from build123d import *

# Parameters (mm, degrees)
F1_DEPTH = 2.54
F2_COUNT = 6
F4_R     = 6.35
F5_DEPTH = 0.508


# Not quite as in the source:
# - a feature names something its author has since deleted; it is built from what else it names


with BuildPart() as f1:
    # F0 (on Top) → F1 (new body)
    with BuildSketch(Plane.XY):
        with BuildLine():
            Line((11.3864204897, -39.6875), (22.9135888085, -39.6875))
            Line((22.9135888085, -39.6875), (0, 0))
            Line((0, 0), (-22.9135888085, -39.6875))
            Line((-22.9135888085, -39.6875), (-11.3864204897, -39.6875))
            ThreePointArc((-11.3864204897, -39.6875), (-10.9170896872, -39.3739031836), (-11.0272102448, -38.8202897552))
            Line((-11.0272102448, -38.8202897552), (-11.8327897552, -38.0147102448))
            ThreePointArc((-11.8327897552, -38.0147102448), (-11.9429103128, -37.4610968164), (-11.4735795103, -37.1475))
            Line((-11.4735795103, -37.1475), (-1.905, -37.1475))
            ThreePointArc((-1.905, -37.1475), (-0.5579615818, -37.7054615818), (0, -39.0525))
            Line((0, -39.0525), (0, -39.6875))
            Line((0, -39.6875), (11.3864204897, -39.6875))
        make_face()
        with BuildLine():
            ThreePointArc((11.0272102448, -40.5547102448), (10.9170896872, -40.0010968164), (11.3864204897, -39.6875))
            Line((11.3864204897, -39.6875), (0, -39.6875))
            Line((0, -39.6875), (0, -40.3225))
            ThreePointArc((0, -40.3225), (0.5579615818, -41.6695384182), (1.905, -42.2275))
            Line((1.905, -42.2275), (11.4735795103, -42.2275))
            ThreePointArc((11.4735795103, -42.2275), (11.9429103128, -41.9139031836), (11.8327897552, -41.3602897552))
            Line((11.8327897552, -41.3602897552), (11.0272102448, -40.5547102448))
        make_face()
    extrude(amount=F1_DEPTH)


with BuildPart() as f2_1:
    # F2: instance of F1
    add(f1.part.rotate(Axis((0, 0, 1.27), (0, 0, -1)), 1 * 360 / F2_COUNT))


with BuildPart() as f2_2:
    # F2: instance of F1
    add(f1.part.rotate(Axis((0, 0, 1.27), (0, 0, -1)), 2 * 360 / F2_COUNT))


with BuildPart() as f2_3:
    # F2: instance of F1
    add(f1.part.rotate(Axis((0, 0, 1.27), (0, 0, -1)), 3 * 360 / F2_COUNT))


with BuildPart() as f2_4:
    # F2: instance of F1
    add(f1.part.rotate(Axis((0, 0, 1.27), (0, 0, -1)), 4 * 360 / F2_COUNT))


with BuildPart() as f2_5:
    # F2: instance of F1
    add(f1.part.rotate(Axis((0, 0, 1.27), (0, 0, -1)), 5 * 360 / F2_COUNT))


with BuildPart() as f1_1:
    add(f1.part)

    # F3: union F2_1, F2_2, F2_3, F2_4, F2_5
    add(f2_1.part)
    add(f2_2.part)
    add(f2_3.part)
    add(f2_4.part)
    add(f2_5.part)

    # F4 (on face) → F5 (cut)
    with BuildSketch(Plane.XY.offset(2.54)):
        with BuildLine():
            Line((13.97, -36.8935), (-13.97, -36.8935))
            Line((-13.97, -36.8935), (-13.97, -39.6875))
            Line((-13.97, -39.6875), (-11.3864204897, -39.6875))
            ThreePointArc((-11.3864204897, -39.6875), (-10.9170896872, -39.3739031836), (-11.0272102448, -38.8202897552))
            Line((-11.0272102448, -38.8202897552), (-11.8327897552, -38.0147102448))
            ThreePointArc((-11.8327897552, -38.0147102448), (-11.9429103128, -37.4610968164), (-11.4735795103, -37.1475))
            Line((-11.4735795103, -37.1475), (-1.905, -37.1475))
            ThreePointArc((-1.905, -37.1475), (-0.5579615818, -37.7054615818), (0, -39.0525))
            Line((0, -39.0525), (0, -40.3225))
            ThreePointArc((0, -40.3225), (0.5579615818, -41.6695384182), (1.905, -42.2275))
            Line((1.905, -42.2275), (11.4735795103, -42.2275))
            ThreePointArc((11.4735795103, -42.2275), (11.9429103128, -41.9139031836), (11.8327897552, -41.3602897552))
            Line((11.8327897552, -41.3602897552), (11.0272102448, -40.5547102448))
            ThreePointArc((11.0272102448, -40.5547102448), (10.9170896872, -40.0010968164), (11.3864204897, -39.6875))
            Line((11.3864204897, -39.6875), (13.97, -39.6875))
            Line((13.97, -39.6875), (13.97, -36.8935))
        make_face()
        with BuildLine():
            Line((-22.9135888085, -39.6875), (-16.5635888085, -39.6875))
            ThreePointArc((-16.5635888085, -39.6875), (-19.7385888085, -34.188238686), (-26.0885888085, -34.188238686))
            Line((-26.0885888085, -34.188238686), (-22.9135888085, -39.6875))
        make_face()
        with BuildLine():
            ThreePointArc((26.0885888085, -34.188238686), (19.7385888085, -34.188238686), (16.5635888085, -39.6875))
            Line((16.5635888085, -39.6875), (22.9135888085, -39.6875))
            Line((22.9135888085, -39.6875), (26.0885888085, -34.188238686))
        make_face()
        with BuildLine():
            Line((-28.6771729679, -29.7046794022), (-27.3853832127, -31.9421248909))
            Line((-27.3853832127, -31.9421248909), (-24.9657082345, -30.5451248909))
            Line((-24.9657082345, -30.5451248909), (-38.9357082345, -6.3483751091))
            Line((-38.9357082345, -6.3483751091), (-41.3553832127, -7.7453751091))
            Line((-41.3553832127, -7.7453751091), (-40.0635934575, -9.9828205978))
            ThreePointArc((-40.0635934575, -9.9828205978), (-39.5573452468, -10.2324745873), (-39.1329622327, -9.8603006727))
            Line((-39.1329622327, -9.8603006727), (-38.8380996671, -8.7598585968))
            ThreePointArc((-38.8380996671, -8.7598585968), (-38.413716653, -8.3876846821), (-37.9074684422, -8.6373386717))
            Line((-37.9074684422, -8.6373386717), (-33.1231786871, -16.9239716058))
            ThreePointArc((-33.1231786871, -16.9239716058), (-32.9328683822, -18.3695218867), (-33.8204570813, -19.52625))
            Line((-33.8204570813, -19.52625), (-34.9203093441, -20.16125))
            ThreePointArc((-34.9203093441, -20.16125), (-35.8078980432, -21.3179781133), (-35.6175877383, -22.7635283942))
            Line((-35.6175877383, -22.7635283942), (-30.8332979832, -31.0501613283))
            ThreePointArc((-30.8332979832, -31.0501613283), (-30.3270497724, -31.2998153179), (-29.9026667583, -30.9276414032))
            Line((-29.9026667583, -30.9276414032), (-29.6078041927, -29.8271993273))
            ThreePointArc((-29.6078041927, -29.8271993273), (-29.1834211786, -29.4550254127), (-28.6771729679, -29.7046794022))
        make_face()
        with BuildLine():
            Line((24.9657082345, -30.5451248909), (27.3853832127, -31.9421248909))
            Line((27.3853832127, -31.9421248909), (28.6771729679, -29.7046794022))
            ThreePointArc((28.6771729679, -29.7046794022), (28.6402555596, -29.1414285963), (28.1057519878, -28.9599890825))
            Line((28.1057519878, -28.9599890825), (27.005309912, -29.254851648))
            ThreePointArc((27.005309912, -29.254851648), (26.4708063402, -29.0734121342), (26.4338889319, -28.5101613283))
            Line((26.4338889319, -28.5101613283), (31.2181786871, -20.2235283942))
            ThreePointArc((31.2181786871, -20.2235283942), (32.3749068004, -19.3359396951), (33.8204570813, -19.52625))
            Line((33.8204570813, -19.52625), (34.9203093441, -20.16125))
            ThreePointArc((34.9203093441, -20.16125), (36.365859625, -20.3515603049), (37.5225877383, -19.4639716058))
            Line((37.5225877383, -19.4639716058), (42.3068774935, -11.1773386717))
            ThreePointArc((42.3068774935, -11.1773386717), (42.2699600852, -10.6140878658), (41.7354565134, -10.432648352))
            Line((41.7354565134, -10.432648352), (40.6350144376, -10.7275109175))
            ThreePointArc((40.6350144376, -10.7275109175), (40.1005108658, -10.5460714037), (40.0635934575, -9.9828205978))
            Line((40.0635934575, -9.9828205978), (41.3553832127, -7.7453751091))
            Line((41.3553832127, -7.7453751091), (38.9357082345, -6.3483751091))
            Line((38.9357082345, -6.3483751091), (24.9657082345, -30.5451248909))
        make_face()
        with BuildLine():
            Line((-45.8271776169, 0), (-42.6521776169, -5.499261314))
            ThreePointArc((-42.6521776169, -5.499261314), (-40.3279163029, -3.175), (-39.4771776169, 0))
            ThreePointArc((-39.4771776169, 0), (-40.3279163029, 3.175), (-42.6521776169, 5.499261314))
            Line((-42.6521776169, 5.499261314), (-45.8271776169, 0))
        make_face()
        with BuildLine():
            ThreePointArc((42.6521776169, 5.499261314), (39.4771776169, 0), (42.6521776169, -5.499261314))
            Line((42.6521776169, -5.499261314), (45.8271776169, 0))
            Line((45.8271776169, 0), (42.6521776169, 5.499261314))
        make_face()
        with BuildLine():
            Line((-40.0635934575, 9.9828205978), (-41.3553832127, 7.7453751091))
            Line((-41.3553832127, 7.7453751091), (-38.9357082345, 6.3483751091))
            Line((-38.9357082345, 6.3483751091), (-24.9657082345, 30.5451248909))
            Line((-24.9657082345, 30.5451248909), (-27.3853832127, 31.9421248909))
            Line((-27.3853832127, 31.9421248909), (-28.6771729679, 29.7046794022))
            ThreePointArc((-28.6771729679, 29.7046794022), (-28.6402555596, 29.1414285963), (-28.1057519878, 28.9599890825))
            Line((-28.1057519878, 28.9599890825), (-27.005309912, 29.254851648))
            ThreePointArc((-27.005309912, 29.254851648), (-26.4708063402, 29.0734121342), (-26.4338889319, 28.5101613283))
            Line((-26.4338889319, 28.5101613283), (-31.2181786871, 20.2235283942))
            ThreePointArc((-31.2181786871, 20.2235283942), (-32.3749068004, 19.3359396951), (-33.8204570813, 19.52625))
            Line((-33.8204570813, 19.52625), (-34.9203093441, 20.16125))
            ThreePointArc((-34.9203093441, 20.16125), (-36.365859625, 20.3515603049), (-37.5225877383, 19.4639716058))
            Line((-37.5225877383, 19.4639716058), (-42.3068774935, 11.1773386717))
            ThreePointArc((-42.3068774935, 11.1773386717), (-42.2699600852, 10.6140878658), (-41.7354565134, 10.432648352))
            Line((-41.7354565134, 10.432648352), (-40.6350144376, 10.7275109175))
            ThreePointArc((-40.6350144376, 10.7275109175), (-40.1005108658, 10.5460714037), (-40.0635934575, 9.9828205978))
        make_face()
        with BuildLine():
            Line((38.9357082345, 6.3483751091), (41.3553832127, 7.7453751091))
            Line((41.3553832127, 7.7453751091), (40.0635934575, 9.9828205978))
            ThreePointArc((40.0635934575, 9.9828205978), (39.5573452468, 10.2324745873), (39.1329622327, 9.8603006727))
            Line((39.1329622327, 9.8603006727), (38.8380996671, 8.7598585968))
            ThreePointArc((38.8380996671, 8.7598585968), (38.413716653, 8.3876846821), (37.9074684422, 8.6373386717))
            Line((37.9074684422, 8.6373386717), (33.1231786871, 16.9239716058))
            ThreePointArc((33.1231786871, 16.9239716058), (32.9328683822, 18.3695218867), (33.8204570813, 19.52625))
            Line((33.8204570813, 19.52625), (34.9203093441, 20.16125))
            ThreePointArc((34.9203093441, 20.16125), (35.8078980432, 21.3179781133), (35.6175877383, 22.7635283942))
            Line((35.6175877383, 22.7635283942), (30.8332979832, 31.0501613283))
            ThreePointArc((30.8332979832, 31.0501613283), (30.3270497724, 31.2998153179), (29.9026667583, 30.9276414032))
            Line((29.9026667583, 30.9276414032), (29.6078041927, 29.8271993273))
            ThreePointArc((29.6078041927, 29.8271993273), (29.1834211786, 29.4550254127), (28.6771729679, 29.7046794022))
            Line((28.6771729679, 29.7046794022), (27.3853832127, 31.9421248909))
            Line((27.3853832127, 31.9421248909), (24.9657082345, 30.5451248909))
            Line((24.9657082345, 30.5451248909), (38.9357082345, 6.3483751091))
        make_face()
        with BuildLine():
            Line((-22.9135888085, 39.6875), (-26.0885888085, 34.188238686))
            ThreePointArc((-26.0885888085, 34.188238686), (-19.7385888085, 34.188238686), (-16.5635888085, 39.6875))
            Line((-16.5635888085, 39.6875), (-22.9135888085, 39.6875))
        make_face()
        with BuildLine():
            ThreePointArc((16.5635888085, 39.6875), (19.7385888085, 34.188238686), (26.0885888085, 34.188238686))
            Line((26.0885888085, 34.188238686), (22.9135888085, 39.6875))
            Line((22.9135888085, 39.6875), (16.5635888085, 39.6875))
        make_face()
        with BuildLine():
            Line((-11.3864204897, 39.6875), (-13.97, 39.6875))
            Line((-13.97, 39.6875), (-13.97, 36.8935))
            Line((-13.97, 36.8935), (13.97, 36.8935))
            Line((13.97, 36.8935), (13.97, 39.6875))
            Line((13.97, 39.6875), (11.3864204897, 39.6875))
            ThreePointArc((11.3864204897, 39.6875), (10.9170896872, 39.3739031836), (11.0272102448, 38.8202897552))
            Line((11.0272102448, 38.8202897552), (11.8327897552, 38.0147102448))
            ThreePointArc((11.8327897552, 38.0147102448), (11.9429103128, 37.4610968164), (11.4735795103, 37.1475))
            Line((11.4735795103, 37.1475), (1.905, 37.1475))
            ThreePointArc((1.905, 37.1475), (0.5579615818, 37.7054615818), (0, 39.0525))
            Line((0, 39.0525), (0, 40.3225))
            ThreePointArc((0, 40.3225), (-0.5579615818, 41.6695384182), (-1.905, 42.2275))
            Line((-1.905, 42.2275), (-11.4735795103, 42.2275))
            ThreePointArc((-11.4735795103, 42.2275), (-11.9429103128, 41.9139031836), (-11.8327897552, 41.3602897552))
            Line((-11.8327897552, 41.3602897552), (-11.0272102448, 40.5547102448))
            ThreePointArc((-11.0272102448, 40.5547102448), (-10.9170896872, 40.0010968164), (-11.3864204897, 39.6875))
        make_face()
        Circle(F4_R)
    extrude(amount=-F5_DEPTH, mode=Mode.SUBTRACT)


solid = f1_1.part
Could you check a few things on this model? Use its own coordinates, in mm. A direction names the side the tool comes from. Round coordinates to 2 decimals unless told otherwise and drop trailing zeros. Write each loop counter-clockwise with the first axis right and the second up, starting at its lowest first coordinate (ties: lowest second). Pieces come first, ordered by that corner, then holes. Notation, with made-up numbers: (9, -37.75) - (15, -37.75) arc R18 ccw to (15, -33.75) - close; hole circle Ø8 at (5.25, -29.75). An arc over 180 degrees is marked (long way). Use a Markdown table: item, result.
Q1. For faces 1 (the flat face through (-42.905, 5.061, 0.97)), 2 (the flat face through (-43, 0, 2.032)), 3 (the flat face through (43, 0, 2.032)), 4 (the cylindrical face through (19.658, 34.235, 2.29)), which set-ups out of +Z, -Z, +X, -X, +Y, -Y let a thin tool reach every point of the face, with its end or its side?
Output values:
| item | result |
|---|---|
| face 1 | +Z, -Z, -X |
| face 2 | +Z, -X |
| face 3 | +Z, +X |
| face 4 | +Z, +Y |
Q2. For pin 1 (0.6 mm diameter, centred on y = 38.5, z = 2.5, fed in from -X); pin 2 (1.5 mm diameter, centred on y = -23.5, z = 0.5, fed in from +X); pin 3 (0.6 mm diameter, centred on y = 39.5, z = 1, fed in from +X), each with a flat end and sliding along its axis, tell me the tip position at first contact or that it passes through.
Output values:
| item | result |
|---|---|
| pin 1 | x = -16.74 |
| pin 2 | x = 29.76 |
| pin 3 | x = 23.2 |
Q3. Please list where these lines run through material, in increasing order: L1, parallel to Y at x = 0, z = 2.3; L2, parallel to Y at x = -11, z = 1.55; L3, parallel to Y at x = 21.5, z = 1.1.
Output values:
| item | result |
|---|---|
| L1 | -36.89 to -6.35, 6.35 to 36.89 |
| L2 | -39.51 to -38.85, -37.15 to 39.87, 40.53 to 42.23 |
| L3 | -39.69 to 39.69 |
Q4. I want a section at A-A (x = -20.5). List the corners of the cut face in (y, z) for me.
Output values:
| item | result |
|---|---|
| outline | (-39.69, 0) - (39.69, 0) - (39.69, 2.03) - (33.81, 2.03) - (33.81, 2.54) - (-33.81, 2.54) - (-33.81, 2.03) - (-39.69, 2.03) - close |
Q5. I want a section at B-B (y = 27). List the corners of the cut face in (x, z) for me, plus the area to 3 significant figures.
Output values:
| item | result |
|---|---|
| outline | (-27.31, 0) - (33.17, 0) - (33.17, 2.03) - (27.01, 2.03) - (27.01, 2.54) - (-27.01, 2.54) - (-27.01, 2.03) - (-27.31, 2.03) - close |
| area | 150 mm2 |
